Autodesk Inventor part; units mm, degrees
ref_plane "Plano de trabalho1" through (0.0009, 0, 0) normal (0, -1, 0) x (1, 0, 0)
ref_plane "YZ Plane" through (0, 0, 0) normal (1, 0, 0) x (0, 1, 0)
ref_plane "XZ Plane" through (0, 0, 0) normal (0, 1, 0) x (-1, 0, 0)
sketch "Esboço1" plane through (0, 0, 0) normal (0, 0, 1) x (1, 0, 0)
  line L0 (25.0389, 40) -> (25.0389, 33.2076)
  line L1 (25.0389, 0) -> (25.0389, 6.7924)
  arc A0 (25.0389, 33.2076) -> (25.0389, 6.7924) centre (48.5809, 20) ccw
  line L2 (24.0389, 0) -> (24.0389, 6.5336)
  line L3 (24.0009, 34.5359) -> (24.0009, 39.0029)
  line L4 (24.0009, 40) -> (25.0389, 40)
  line L5 (24.0389, 33.4664) -> (5.7012, 33.4664)
  line L6 (5.6632, 34.5359) -> (24.0009, 34.5359)
  line L7 (24.0009, 39.0029) -> (24.0009, 40)
  line L8 (5.6632, 34.5359) -> (4.6632, 34.5359)
  line L9 (5.7012, 33.4664) -> (4.7012, 33.4664)
  line L10 (25.0389, 0) -> (24.0389, 0)
  line L11 (24.0009, 34.5359) -> (0.0009, 34.5359)
  line L12 (4.7012, 33.4664) -> (0.0389, 33.4664)
  line L13 (0.0009, 34.5359) -> (0.0009, -0.006)
  line L14 (0.0009, 6.5336) -> (0.0009, 7.5336)
  line L15 (0.0009, 6.5336) -> (0.0009, 7.5336)
  line L16 (0.0009, 6.5336) -> (0.0009, 7.5336)
  line L17 (0.0009, 6.5336) -> (0.0009, 7.5336)
  line L18 (0.0009, 34.5359) -> (0.0009, 33.4664)
  line L19 (0.0389, 33.4664) -> (0.0009, 33.4664)
  line L20 (22.7806, 9.1373) -> (0.0009, 9.1373)
  line L21 (0.0009, 8.062) -> (23.2602, 8.062)
  line L22 (23.5161, 7.5336) -> (24.0389, 6.5336)
  arc A1 (24.0389, 33.4664) -> (22.7806, 9.1373) centre (48.5809, 20) ccw
  arc A2 (23.2602, 8.062) -> (23.5161, 7.5336) centre (48.5809, 20) ccw
  line L23 (0.0009, 9.1373) -> (0.0009, 8.062)
  line L24 (0.0009, 8.062) -> (0.0009, 7.062)
  point P0 (0, 0)
  point P1 (0, 0)
  point P2 (0.0199, 33.4664)
  dimension "d16" = 24.3291
  dimension "d17" = 1.0695
  dimension "d19" = 1
revolve "Revolução1" add sketch "Esboço1" angle 360 about axis through (0.0009, 34.5359, 0) along (0, -1, 0) contours L0 A0 L1 L10 L2 L22 A2 L21 L13 L20 A1 L5 L9 L12 L19 L11 L8 L6 L3 L7 L4
sketch "Esboço2" plane through (0.0009, 8.062, 0) normal (0, -1, 0) x (1, 0, 0)
  point P0 (-0.0009, 0)
sketch "Esboço3" plane through (0.0009, 34.5359, 0) normal (0, 1, 0) x (1, 0, 0)
  circle A0 centre (-0.0009, 0) radius 3.5
  circle A1 centre (-0.0009, 0) radius 17.1056
  line L0 (-0.0009, 0) -> (-7.5211, 15.3639)
  line L1 (-0.0009, 0) -> (-0.0009, 6.0664)
  line L2 (-0.0009, 0) -> (7.5193, 15.3639)
  line L3 (-0.0009, 0) -> (-15.3648, -7.5202)
  line L4 (-0.0009, 0) -> (-15.3648, 7.5202)
  line L5 (-0.0009, 0) -> (7.5193, -15.3639)
  line L6 (-0.0009, 0) -> (-7.5211, -15.3639)
  line L7 (-0.0009, 0) -> (15.3629, 7.5202)
  line L8 (-0.0009, 0) -> (15.3629, -7.5202)
  point P0 (-3.1445, 1.5387)
  point P1 (-3.1445, -1.5387)
  point P2 (3.1427, -1.5387)
  point P3 (3.1427, 1.5387)
  point P4 (-1.5396, -3.1436)
  point P5 (1.5378, -3.1436)
  point P6 (1.5378, 3.1436)
  point P7 (-1.5396, 3.1436)
  dimension "d1" = 7
  dimension "d4" = 360
extrude "Extrusão1" cut sketch "Esboço3" against normal blind 10 contours A0 L7 A1 L8 | A0 L0 A1 L2 | L5 A1 L6 A0 | L3 A1 L4 A0
sketch "Esboço4" plane through (0.0009, 8.062, 0) normal (0, -1, 0) x (1, 0, 0)
  circle A0 centre (-0.0009, 0) radius 1.5
  circle A1 centre (-0.0009, 6.6683) radius 1.5
  line L0 (-0.0009, 0) -> (-5.2667, 0)
  circle A2 centre (-0.0009, -6.6683) radius 1.5
  dimension "d8" = 3
  dimension "d9" = 3
extrude "Extrusão2" cut sketch "Esboço4" against normal blind 10
ref_plane "Plano de trabalho1" through (0.0009, 0, 0) normal (0, -1, 0) x (1, 0, 0)
sketch "Esboço5" plane through (0.0009, 0, 0) normal (0, -1, 0) x (1, 0, 0)
  circle A0 centre (0, 0) radius 25.038
  line L0 (0, 25.038) -> (0, 27.459) construction
  line L1 (-2.4513, 25.038) -> (-2.4513, 27.459)
  line L2 (2.4513, 27.459) -> (2.4513, 25.038)
  arc A1 (2.4513, 27.459) -> (-2.4513, 27.459) centre (0, 27.459) ccw
  line L3 (-7.3697, 0) -> (-12.5067, 0)
  circle A2 centre (0, 27.459) radius 1.4892
  line L4 (-2.4513, -25.038) -> (-2.4513, -27.459)
  line L5 (2.4513, -27.459) -> (2.4513, -25.038)
  arc A3 (-2.4513, -27.459) -> (2.4513, -27.459) centre (0, -27.459) ccw
  circle A4 centre (0, -27.459) radius 1.4892
  arc A5 (-2.4513, 25.038) -> (-2.4484, 24.918) centre (0, 25.038) ccw
  arc A6 (2.4484, 24.918) -> (2.4513, 25.038) centre (0, 25.038) ccw
  arc A7 (2.4513, -25.038) -> (2.4484, -24.918) centre (0, -25.038) ccw
  arc A8 (-2.4484, -24.918) -> (-2.4513, -25.038) centre (0, -25.038) ccw
  point P0 (-0.0009, 0)
  point P1 (0, 26.2485)
  dimension "d15" = 2.9784
extrude "Extrusão3" add sketch "Esboço5" against normal blind 1 contours A0 A5 L1 A1 L2 A6 | A7 L5 A3 L4 A8 A0
properties part number "acoplamento_ventoinha1"
The model under review builds one solid part; all positions refer to its coordinate system, in mm. A direction names the side the tool comes from. Round coordinates to 2 decimals unless told otherwise and drop trailing zeros. Order: outer loops, then holes, each group sorted by start corner. A loop starts at its lowest first (then second) coordinate and runs counter-clockwise, first axis right, second up.
(1) For P1, Ø6, axis at x = -3, y = 35, coming from the +Z side; P2, Ø1.5, axis at x = -11, z = -15.5, coming from the +Y side; P3, Ø1.8, axis at x = 0, z = -27.46, coming from the -Y side; P4, Ø6, axis at x = 10, y = 28, coming from the +Z side, all flat-tipped, find the tip position at first contact; note any pin that passes through.
Working result:
P1: stops at z = 25.04
P2: stops at y = 34.54
P3: passes through
P4: stops at z = 22.21
(2) Tool access review of faces 1 (the face through (-9.17, 34.01, 4.49)), 2 (the face through (-1.5, 8.59, 0.07)), 3 (the face through (-0.322, 0.493, -28.913)): name each direction out of +Z, -Z, +X, -X, +Y, -Y from which nothing blocks a thin tool from reaching the whole face with its end or side.
Working result:
face 1: +Y
face 2: -Y
face 3: +Y, -Y
(3) Wall thickness on L1, parallel to Y at x = -0.5, z = 2.5; L2, parallel to Y at x = 21.5, z = -9.5; L3, parallel to X at y = 13, z = 13.5: over which ranges is each line inside the solid? List them lowest first.
Working result:
L1: y = 8.06 to 9.14, 33.47 to 34.54
L2: y = 7.56 to 10.01, 29.99 to 32.44, 33.47 to 34.54
L3: x = -18.01 to -16.7, 16.7 to 18.01
(4) Mouldability with a two-part tool opening along Z and no side actions: class faces 4 (the face through (13.461, 3.444, -21.112)), 5 (the face through (-4.49, 34.01, 9.17)), 6 (the face through (-0.05, 0.49, -29.91)), 7 (the face through (-23.976, 37.306, -1.055)) as released by +Z, released by -Z, zero draft, split by the parting line, or undercut.
Working result:
face 4: split by the parting line
face 5: undercut
face 6: released by -Z
face 7: undercut
(5) Take a section at A-A, the plane x = 0. Count the separate pieces of the cut face and the enclosed holes in it, plus the area to 3 significant figures.
Working result:
separate pieces: 7
enclosed holes: 0
area: 149 mm2
(6) Take a section at C-C, the plane y = 22. State the section outline as (x, z) points, plus the area to 3 significant figures.
Working result:
outline: circle Ø43.32 at (0, 0); hole circle Ø41.32 at (0, 0)
area: 133 mm2
